Study the drawing (mm; zero at the part's minimum x, y, z) and answer. Give positions to 0.01 mm unless a question says otherwise; leave off trailing zeros. Write each loop counter-clockwise with the first axis right and the second up, starting at its lowest first coordinate (ties: lowest second). Pieces come first, ordered by that corner, then holes.
1) Given pin 1 Ø6 at (y, z) = (15.5, 68.5) entering from +X; pin 2 Ø2 at (y, z) = (20, 32.5) entering from -X, each flat-ended and moving along its own axis, determine where each tip first touches the part or whether it passes through.
2) Find section C-C (y = 23.5). Determine the outline of the cut face in (x, z), plus the area to 3 significant figures.
3) Straight lines are drawn through the part: probe 1 along X at (y, z) = (20.5, 85.5); probe 2 along Z at (x, y) = (118, 6). For each, find the intervals that lie inside material, in ascending order.
4) Determine the mould class of the marked faces 1, 2 and 3 for opening direction Z: pulls with the +Z half, pulls with the -Z half, needs draft (parallel to the pull), parting line crosses it, or undercut.
5) Find section D-D (z = 37.5). Determine the outline of the cut face in (x, y).
6) Find section A-A (y = 5.08). Determine the outline of the cut face in (x, z) (3 decimals), plus the area to 3 significant figures.
7) Find section B-B (z = 121.92). Determine the outline of the cut face in (x, y) (3 decimals), plus the area to 3 significant figures.
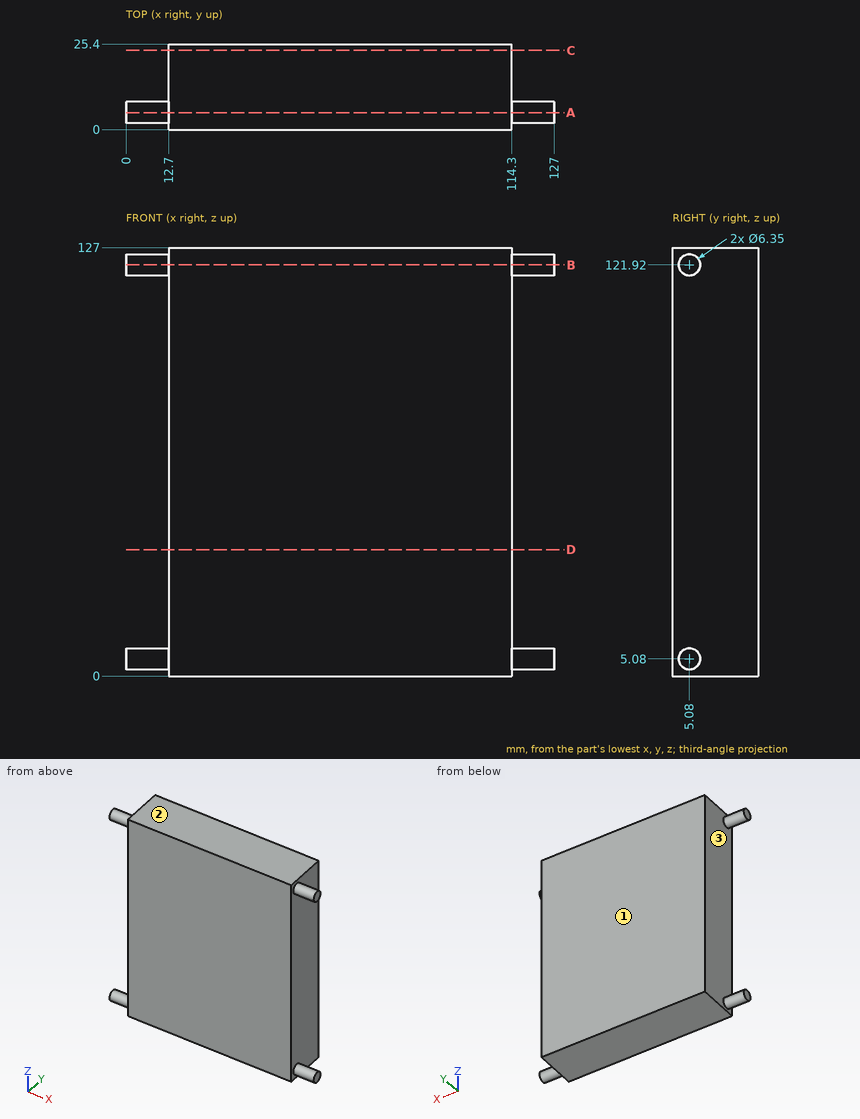
Results:
1. pin 1: stops at x = 114.3
1. pin 2: stops at x = 12.7
2. outline: (12.7, 0) - (114.3, 0) - (114.3, 127) - (12.7, 127) - close
2. area: 12,900 mm2
3. probe 1: x = 12.7 to 114.3
3. probe 2: z = 2.04 to 8.12, 118.88 to 124.96
4. face 1: needs draft
4. face 2: pulls with the +Z half
4. face 3: undercut
5. outline: (12.7, 0) - (114.3, 0) - (114.3, 25.4) - (12.7, 25.4) - close
6. outline: (0, 1.905) - (12.7, 1.905) - (12.7, 0) - (114.3, 0) - (114.3, 1.905) - (127, 1.905) - (127, 8.255) - (114.3, 8.255) - (114.3, 118.745) - (127, 118.745) - (127, 125.095) - (114.3, 125.095) - (114.3, 127) - (12.7, 127) - (12.7, 125.095) - (0, 125.095) - (0, 118.745) - (12.7, 118.745) - (12.7, 8.255) - (0, 8.255) - close
6. area: 13,200 mm2
7. outline: (0, 1.905) - (12.7, 1.905) - (12.7, 0) - (114.3, 0) - (114.3, 1.905) - (127, 1.905) - (127, 8.255) - (114.3, 8.255) - (114.3, 25.4) - (12.7, 25.4) - (12.7, 8.255) - (0, 8.255) - close
7. area: 2,740 mm2
